Verification items for this drawing (mm, ordinates from the low corner). A direction names the side the tool comes from. Give positions to 0.01 mm unless a question says otherwise; leave off trailing zeros. Loops run counter-clockwise (first coordinate to the right, second up) from the corner with the lowest first, then second, coordinate; pieces in that order, holes last. Notation, with made-up numbers: (25.25, -10.5) -> (64.25, -10.5) arc R13 cw to (64.25, 6.5) -> close; hole circle Ø2 at (75, 64.5). An arc over 180 degrees is marked (long way). Answer as CSV lines item,"result". Start each with the question number.
(1) Section check B-B on z = 3.75. Enter the section's corners in (x, y), plus the area to 3 significant figures.
(2) Section check D-D on y = 7.75. Enter the section's corners in (x, z), plus the area to 3 significant figures.
(3) Material ranges on line 1 (Z direction, x = 3, y = 1.5); line 2 (X direction, y = 6.75, z = 6); line 3 (Y direction, x = 8, z = 4.25), recorded low to high. Write a range as from..to.
(4) Section check A-A on x = 3. Enter the section's corners in (y, z).
(5) Access from +Z, -Z, +X, -X, +Y, -Y to the whole of each face (thin tool, end or side, straight path). Record for the marked faces 4, 5 and 6.
(6) Gauge pin test, flat ends, axial feed: pin 1 Ø4 at (y, z) = (8.5, 6) entering from -X; pin 2 Ø1.5 at (x, z) = (13.5, 2.5) entering from +Y; pin 3 Ø6 at (x, y) = (23, 4.5) entering from -Z; pin 4 Ø4 at (x, z) = (5.5, 4.5) entering from +Y. Record the tip position at first contact, or that the pin passes through.
(7) Section check C-C on x = 16.5. Enter the section's corners in (y, z).
(8) Release check for a two-part mould opening along X. For the marked faces 1, 2 and 3 record: pulls with the +X half, pulls with the -X half, needs draft (parallel to the pull), parting line crosses it, or undercut.
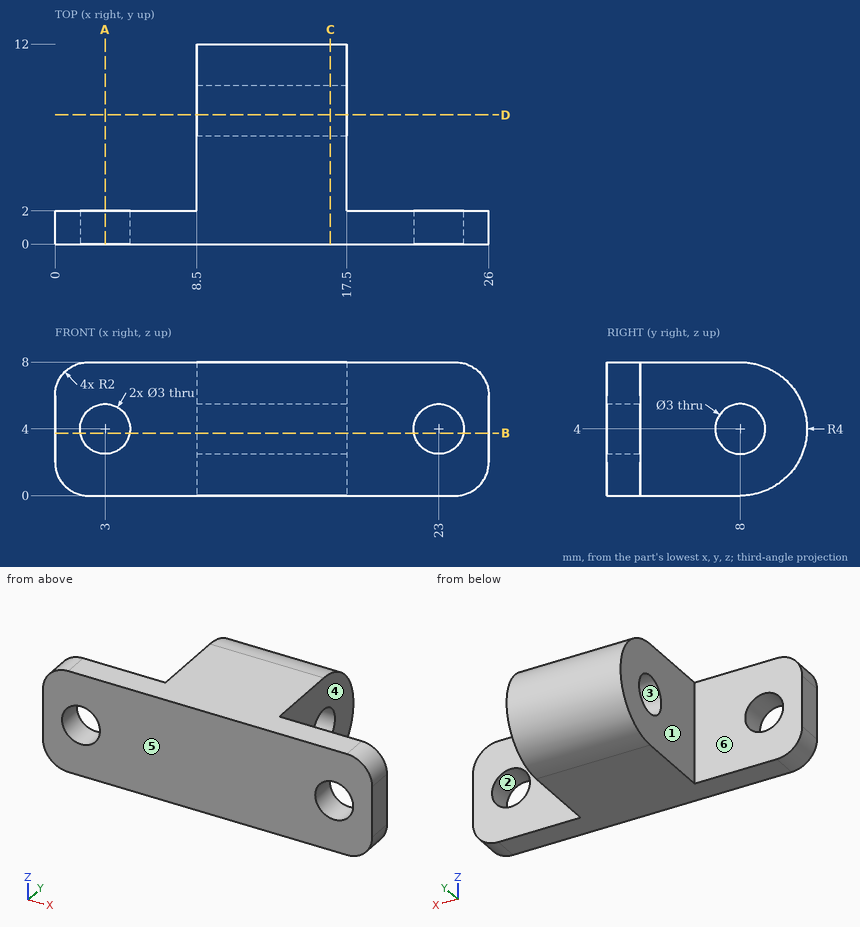
Working result:
1,outline,"(0, 0) -> (1.52, 0) -> (1.52, 2) -> (0, 2) -> close; (4.48, 0) -> (21.52, 0) -> (21.52, 2) -> (17.5, 2) -> (17.5, 6.52) -> (8.5, 6.52) -> (8.5, 2) -> (4.48, 2) -> close; (8.5, 9.48) -> (17.5, 9.48) -> (17.5, 11.99) -> (8.5, 11.99) -> close; (24.48, 0) -> (26, 0) -> (26, 2) -> (24.48, 2) -> close"
1,area,"103 mm^2"
2,outline,"(8.5, 0) -> (17.5, 0) -> (17.5, 2.52) -> (8.5, 2.52) -> close; (8.5, 5.48) -> (17.5, 5.48) -> (17.5, 8) -> (8.5, 8) -> close"
2,area,"45.4 mm^2"
3,line 1,"z = 0..2.5, 5.5..8"
3,line 2,"x = 8.5..17.5"
3,line 3,"y = 0..2"
4,outline,"(0, 0) -> (2, 0) -> (2, 2.5) -> (0, 2.5) -> close; (0, 5.5) -> (2, 5.5) -> (2, 8) -> (0, 8) -> close"
5,face 4,"+Z, -Z, +X, +Y"
5,face 5,"+Z, -Z, +X, -X, -Y"
5,face 6,"+Z, -Z, -X, +Y"
6,pin 1,"stops at x = 8.5"
6,pin 2,"stops at y = 11.93"
6,pin 3,"stops at z = 0"
6,pin 4,"stops at y = 2"
7,outline,"(0, 0) -> (8, 0) arc R4 ccw to (8, 8) -> (0, 8) -> close; hole circle Ø3 at (8, 4)"
8,face 1,"pulls with the -X half"
8,face 2,"undercut"
8,face 3,"needs draft"
